Could you check a few things on this drawing? It's one solid part, dimensions in mm from its lowest x, y, z. A direction names the side the tool comes from. Give positions to 0.01 mm unless a question says otherwise; leave off trailing zeros. Loops run counter-clockwise (first coordinate to the right, second up) from the corner with the lowest first, then second, coordinate; pieces in that order, holes last. Notation, with made-up numbers: (62.25, -37.75) -> (119.25, -37.75) arc R15 cw to (119.25, -17.75) -> close; hole circle Ø4 at (-23, -10). An arc over 180 degrees is marked (long way). One line per question, with ' | ' between items.
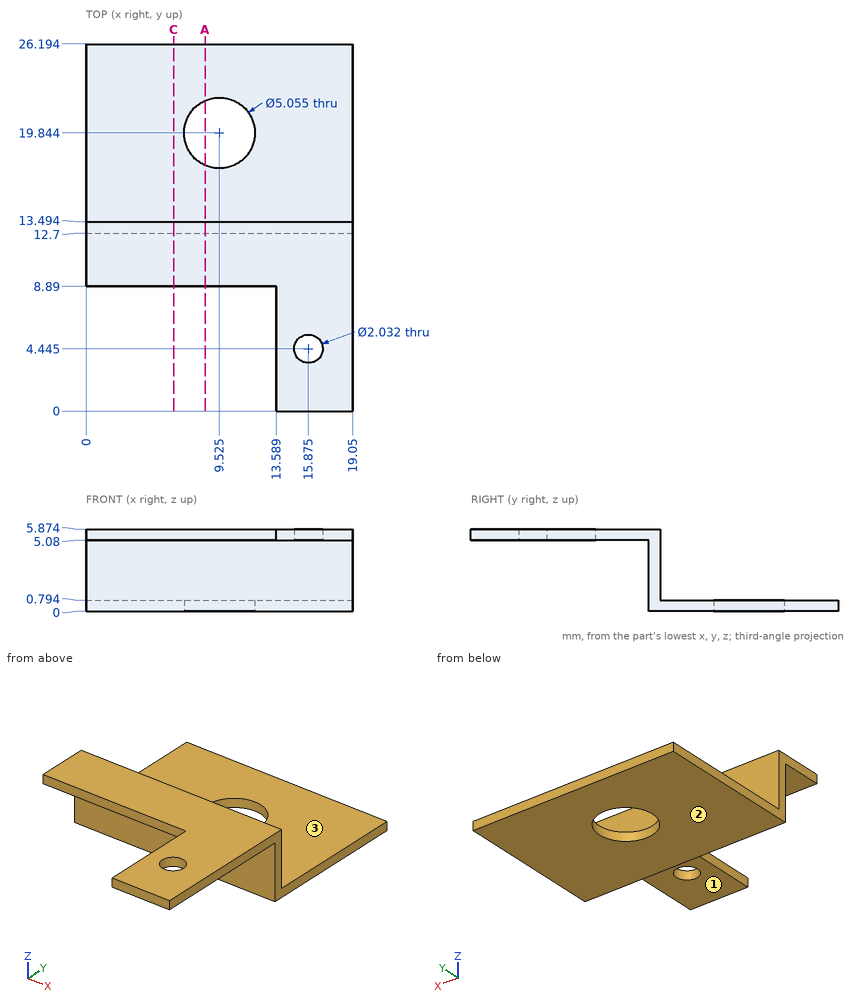
Q1. For pin 1 Ø8 at (x, y) = (9.52, 19.84) entering from -Z; pin 2 Ø1 at (x, z) = (6.5, 0.5) entering from -Y; pin 3 Ø10 at (x, y) = (8, 5.5) entering from -Z; pin 4 Ø4 at (x, y) = (14, 18) entering from +Z, each with a flat end and sliding along its axis, tell me the tip position at first contact or that it passes through.
Entries:
pin 1: z = 0 | pin 2: y = 12.7 | pin 3: z = 5.08 | pin 4: z = 0.79
Q2. On a 3-axis mill with a long thin cutter (end or side, diameter ignored), from which of +Z, -Z, +X, -X, +Y, -Y can I reach the whole of each face in a straight line? I mean the marked faces 1, 2 and 3. Say none if no direction works.
Entries:
face 1: -Z, +X, -X, -Y | face 2: -Z, +X, -X, +Y, -Y | face 3: +Z, +X, -X, +Y
Q3. If we section it at A-A (x = 8.5): Write out the boundary of the cut face in (y, z), plus the area to 3 significant figures.
Entries:
outline: (8.89, 5.08) -> (12.7, 5.08) -> (12.7, 0) -> (17.53, 0) -> (17.53, 0.79) -> (13.49, 0.79) -> (13.49, 5.87) -> (8.89, 5.87) -> close; (22.15, 0) -> (26.19, 0) -> (26.19, 0.79) -> (22.15, 0.79) -> close | area: 14.1 mm²
Q4. If I drill on probe 1 along Z at (x, y) = (16.25, 2.75); probe 2 along Z at (x, y) = (5, 24.5); probe 3 along Y at (x, z) = (12.5, 1.6), over which ranges is the centre line in solid material (lowest first)? Write a range as from..to.
Entries:
probe 1: 5.08..5.87 | probe 2: 0..0.79 | probe 3: 12.7..13.49
Q5. If we section it at C-C (x = 6.25): Write out the boundary of the cut face in (y, z).
Entries:
outline: (8.89, 5.08) -> (12.7, 5.08) -> (12.7, 0) -> (26.19, 0) -> (26.19, 0.79) -> (13.49, 0.79) -> (13.49, 5.87) -> (8.89, 5.87) -> close
